```python
from build123d import *

# Parameters (mm, degrees)
SKETCH5_W           = 110
SKETCH5_H           = 80
SKETCH5_R           = 1
BOSS_EXTRUDE1_DEPTH = 3
SKETCH6_R           = 1.5
CUT_EXTRUDE1_DEPTH  = 137.047785723
FILLET1_R           = 2.5
CUT_EXTRUDE2_DEPTH  = 6
FILLET2_R           = 5


with BuildPart() as part:
    # Sketch5 → Boss-Extrude1 (new body)
    with BuildSketch(Plane(origin=(0, 0, 0), x_dir=(1, 0, 0), z_dir=(0, 1, 0))):
        with Locations((55, 40)):
            Rectangle(SKETCH5_W, SKETCH5_H)
        with Locations(Location((91.764887736, 67.92075713, 0), (0, 0, 270))):
            Circle(SKETCH5_R, mode=Mode.SUBTRACT)
        with Locations(Location((21.764888364, 59.920762627, 0), (0, 0, 270))):
            Circle(SKETCH5_R, mode=Mode.SUBTRACT)
        with Locations(Location((21.764888364, 19.920762627, 0), (0, 0, 270))):
            Circle(SKETCH5_R, mode=Mode.SUBTRACT)
        with Locations(Location((91.764887736, 11.92075713, 0), (0, 0, 270))):
            Circle(SKETCH5_R, mode=Mode.SUBTRACT)
    extrude(amount=BOSS_EXTRUDE1_DEPTH)

    # Sketch6 → Cut-Extrude1 (cut, through all)
    with BuildSketch(Plane(origin=(0, 3, 0), x_dir=(1, 0, 0), z_dir=(0, 1, 0))):
        with Locations(Location((5, 75, 0), (0, 0, 270))):
            Circle(SKETCH6_R)
        with Locations(Location((105, 75, 0), (0, 0, 270))):
            Circle(SKETCH6_R)
        with Locations(Location((105, 5, 0), (0, 0, 270))):
            Circle(SKETCH6_R)
        with Locations(Location((5, 5, 0), (0, 0, 270))):
            Circle(SKETCH6_R)
    extrude(amount=-CUT_EXTRUDE1_DEPTH, mode=Mode.SUBTRACT)

    # Fillet1
    fillet1_edges = [part.edges().sort_by_distance(p)[0] for p in [
        (0, 1.5, -80),
        (110, 1.5, -80),
        (110, 1.5, 0),
        (0, 1.5, 0),
    ]]
    fillet(fillet1_edges, radius=FILLET1_R)

    # Sketch7 → Cut-Extrude2 (cut)
    with BuildSketch(Plane(origin=(0, 3, 0), x_dir=(1, 0, 0), z_dir=(0, 1, 0))):
        Polygon((78.714883487, -234.464098532), (78.714883487, 0), (78.714883487, 15.270760033), (58.814883708, 15.270760033), (58.814883708, 0), (58.814883708, -234.464098532), (58.814883708, -703.392295596), (78.714883487, -703.392295596), align=None)
    extrude(amount=-CUT_EXTRUDE2_DEPTH, mode=Mode.SUBTRACT)

    # Fillet2
    fillet2_edges = [part.edges().sort_by_distance(p)[0] for p in [
        (78.714883487, 1.5, 0),
        (58.814883708, 1.5, 0),
    ]]
    fillet(fillet2_edges, radius=FILLET2_R)


solid = part.part
```
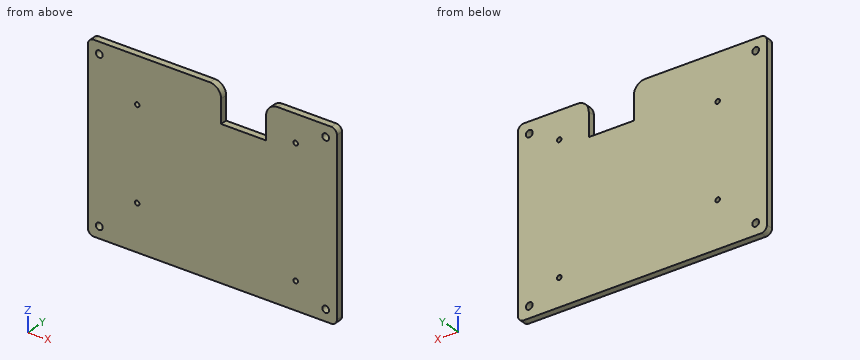
Geometry check sheet. Reference: the model listing, model coordinates, mm. Coordinates: 2 decimals unless noted, no trailing zeros. Loops run counter-clockwise (first coordinate to the right, second up) from the corner with the lowest first, then second, coordinate; pieces in that order, holes last.
Item 1: Sectioned sample at A-A, the plane x = 105. Record the boundary of the cut face in (y, z), then the cut area to 3 significant figures.
Item 2: Thickness scan on line 1 (X direction, y = 1.6, z = -75); line 2 (X direction, y = 1.45, z = -68); line 3 (X direction, y = 0.75, z = -11.5). Record the ranges inside material, lowest first.
Item 3: Sectioned sample at B-B, the plane z = -75. Record the boundary of the cut face in (x, y).
Item 4: Sectioned sample at D-D, the plane x = 75.5. Record the boundary of the cut face in (y, z), then the cut area to 3 significant figures.
Item 5: Sectioned sample at C-C, the plane y = 2.3. Count the separate pieces of the cut face and the enclosed holes in it, then the cut area to 3 significant figures.
Check result:
1. outline: (0, -80) - (3, -80) - (3, -76.5) - (0, -76.5) - close; (0, -73.5) - (3, -73.5) - (3, -6.5) - (0, -6.5) - close; (0, -3.5) - (3, -3.5) - (3, 0) - (0, 0) - close
1. area: 222 mm2
2. line 1: x = 0 to 3.5, 6.5 to 103.5, 106.5 to 110
2. line 2: x = 0 to 90.77, 92.76 to 110
2. line 3: x = 0 to 58.81, 78.71 to 90.86, 92.67 to 110
3. outline: (0, 0) - (3.5, 0) - (3.5, 3) - (0, 3) - close; (6.5, 0) - (103.5, 0) - (103.5, 3) - (6.5, 3) - close; (106.5, 0) - (110, 0) - (110, 3) - (106.5, 3) - close
4. outline: (0, -80) - (3, -80) - (3, -15.27) - (0, -15.27) - close
4. area: 194 mm2
5. separate pieces: 1
5. enclosed holes: 8
5. area: 8,440 mm2
